Read the model definition and answer for the solid it produces. Units are mm, in the model's axes. Face numbers are marked on the shaded views. A direction names the side the tool comes from. Give positions to 0.01 mm unless a question says otherwise; leave off trailing zeros. Write each loop counter-clockwise with the first axis right and the second up, starting at its lowest first coordinate (ties: lowest second). Pieces come first, ordered by that corner, then holes. Notation, with made-up numbers: (60.5, 12) - (116.5, 12) arc R11 cw to (116.5, 20) - close; hole circle Ø5 at (66, 74). An arc over 180 degrees is marked (long way). Answer as a JSON object with one key per item and string values. Group by question number.
```python
from build123d import *

# Parameters (mm, degrees)
BOSS_EXTRUDE1_DEPTH = 5
SKETCH2_W           = 17
SKETCH2_H           = 20
BOSS_EXTRUDE2_DEPTH = 10
SKETCH3_R           = 1
CUT_EXTRUDE1_DEPTH  = 18
SKETCH4_R           = 2.15
CUT_EXTRUDE2_DEPTH  = 6


with BuildPart() as part:
    # Sketch1 → Boss-Extrude1 (new body)
    with BuildSketch(Plane.XY):
        Polygon((-12.102505447, 7.889651416), (11.397494553, 7.889651416), (11.397494553, 27.889651416), (-12.102505447, 27.889651416), (-12.102505447, 26.889651416), (-0.102505447, 26.889651416), (-0.102505447, 22.98867093), (1.897494553, 22.98867093), (1.897494553, 12.790631903), (-0.102505447, 12.790631903), (-0.102505447, 8.889651416), (-1.102505447, 8.889651416), (-12.102505447, 8.889651416), align=None)
    extrude(amount=BOSS_EXTRUDE1_DEPTH)

    # Sketch2 → Boss-Extrude2 (add)
    with BuildSketch(Plane.XY.offset(5)):
        with Locations((-3.602505447, 17.889651416)):
            Rectangle(SKETCH2_W, SKETCH2_H)
    extrude(amount=BOSS_EXTRUDE2_DEPTH)

    # Sketch3 → Cut-Extrude1 (cut, through all)
    with BuildSketch(Plane(origin=(4.897494553, 0, 0), x_dir=(0, 0, -1), z_dir=(1, 0, 0))):
        with Locations((-12, 17.889651416)):
            Circle(SKETCH3_R)
    extrude(amount=-CUT_EXTRUDE1_DEPTH, mode=Mode.SUBTRACT)

    # Sketch4 → Cut-Extrude2 (cut, through all)
    with BuildSketch(Plane.XY.offset(5)):
        with Locations((8.797494553, 12.789651416)):
            Circle(SKETCH4_R)
        with Locations((8.797494553, 22.989651416)):
            Circle(SKETCH4_R)
    extrude(amount=-CUT_EXTRUDE2_DEPTH, mode=Mode.SUBTRACT)


solid = part.part
```
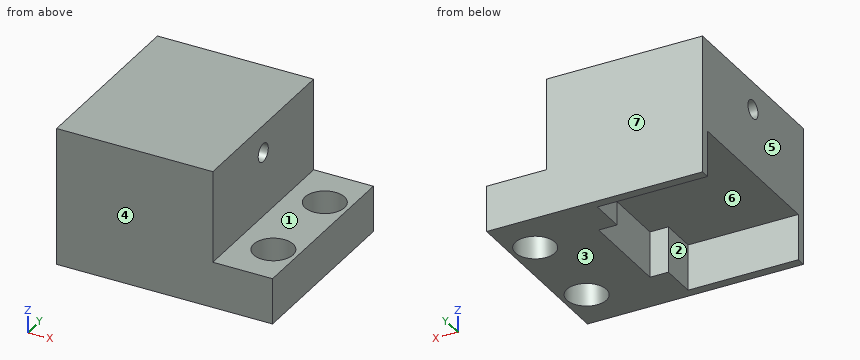
1) Flat-ended cylindrical pins translate along their axes: pin 1 Ø2 at (y, z) = (10.5, 1.5) entering from -X; pin 2 Ø2 at (x, y) = (9, 14) entering from +Z; pin 3 Ø7 at (x, y) = (-7, 21.5) entering from -Z; pin 4 Ø4 at (x, y) = (8.8, 22.99) entering from +Z. Find the tip coordinate at first contact, or state that the pin passes through.
2) Find the intervals of material crossed by line 1 (Y direction, x = -5, z = 2); line 2 (Y direction, x = -2.25, z = 12); line 3 (Z direction, x = -5, y = 21.5), in increasing order. Write a range as [from, to].
3) Find section B-B, the plane x = 8.5. Write down the section's boundary in (y, z).
4) Which of the six approach directions +Z, -Z, +X, -X, +Y, -Y give full straight-line access (tool end or side, diameter ignored) to the marked faces 1, 2 and 3?
5) Find section D-D, the plane y = 10. Write down the section's boundary in (x, z), and give its area (4 significant figures).
6) For a pull along Y with two mould halves and no side action, classify the marked faces 4, 5, 6 and 7 as released by +Y, released by -Y, zero draft, split by the parting line, or undercut.
7) Find section C-C, the plane y = 18.5. Write down the section's boundary in (x, z), and give its area (3 significant figures).
8) Find section A-A, the plane z = 12. Write down the section's boundary in (x, y).
Values follow:
{
 "1": {"pin 1": "stops at x = -0.1", "pin 2": "stops at z = 5", "pin 3": "stops at z = 5", "pin 4": "passes through"},
 "2": {"line 1": "y = [7.89, 8.89], [26.89, 27.89]", "line 2": "y = [7.89, 16.89], [18.89, 27.89]", "line 3": "z = [5, 15]"},
 "3": {"outline": "(7.89, 0) - (10.66, 0) - (10.66, 5) - (7.89, 5) - close; (14.92, 0) - (20.86, 0) - (20.86, 5) - (14.92, 5) - close; (25.12, 0) - (27.89, 0) - (27.89, 5) - (25.12, 5) - close"},
 "4": {"face 1": "+Z, +X, +Y, -Y", "face 2": "-Z, -X", "face 3": "-Z, +X, -X, +Y, -Y"},
 "5": {"outline": "(-12.1, 5) - (-0.1, 5) - (-0.1, 0) - (11.4, 0) - (11.4, 5) - (4.9, 5) - (4.9, 15) - (-12.1, 15) - close", "area": "227.5 mm2"},
 "6": {"face 4": "released by -Y", "face 5": "zero draft", "face 6": "undercut", "face 7": "released by +Y"},
 "7": {"outline": "(-12.1, 5) - (1.9, 5) - (1.9, 0) - (11.4, 0) - (11.4, 5) - (4.9, 5) - (4.9, 11.21) - (-12.1, 11.21) - close; (-12.1, 12.79) - (4.9, 12.79) - (4.9, 15) - (-12.1, 15) - close", "area": "191 mm2"},
 "8": {"outline": "(-12.1, 7.89) - (4.9, 7.89) - (4.9, 16.89) - (-12.1, 16.89) - close; (-12.1, 18.89) - (4.9, 18.89) - (4.9, 27.89) - (-12.1, 27.89) - close"}
}
